The figure shows three views and two pictorial views of one solid part (mm, origin at its lowest corner). Answer the questions. Give positions to 0.01 mm unless a question says otherwise; leave off trailing zeros. Loops run counter-clockwise (first coordinate to the right, second up) from the corner with the lowest first, then second, coordinate; pieces in that order, holes last. Notation, with made-up numbers: M -14.75,53 L 20.25,53 A25 ccw 20.25,71 Z; hole C 0.5,74.25 d7. An arc over 180 degrees is marked long. Answer as a JSON object with one key per item and string values. Group by question number.
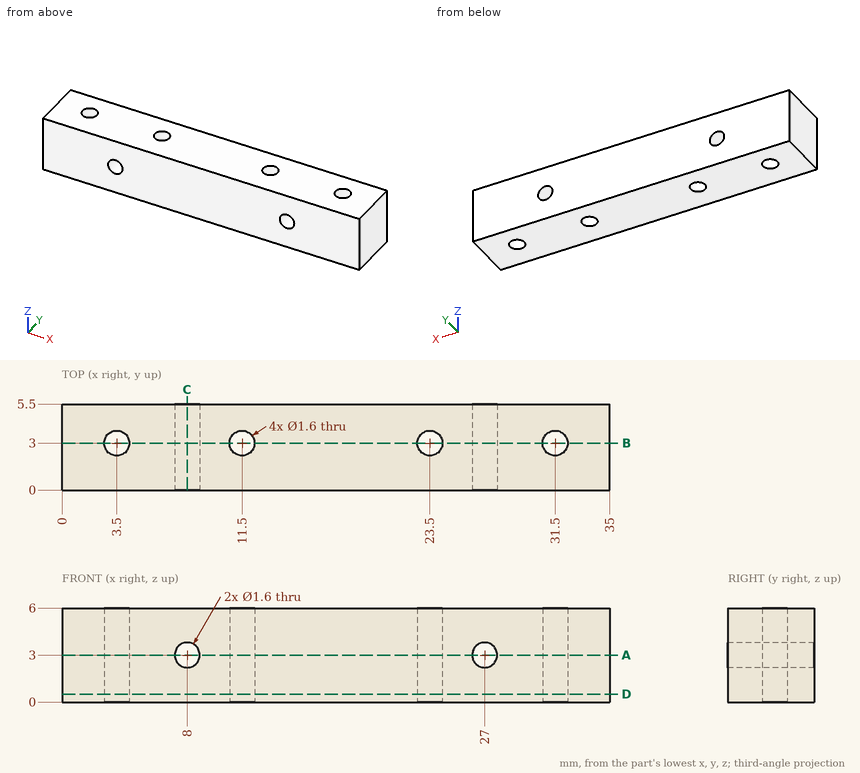
Item 1: A cutting plane is placed at C-C (x = 8). Determine the outline of the cut face in (y, z), and give its area (3 significant figures).
Item 2: Find the intervals of material crossed by probe 1 along Y at (x, z) = (3.5, 4.45); probe 2 along Z at (x, y) = (8, 4.45); probe 3 along X at (y, z) = (0.55, 3.1), in increasing order. Write a range as [from, to].
Item 3: A cutting plane is placed at D-D (z = 0.5). Determine the outline of the cut face in (x, y), and give its area (3 significant figures).
Item 4: A cutting plane is placed at B-B (y = 3). Determine the outline of the cut face in (x, z), and give its area (3 significant figures).
Item 5: A cutting plane is placed at A-A (z = 3). Determine the outline of the cut face in (x, y).
The answers:
{
 "1": {"outline": "M 0,0 L 5.5,0 L 5.5,2.2 L 0,2.2 Z; M 0,3.8 L 5.5,3.8 L 5.5,6 L 0,6 Z", "area": "24.2 mm^2"},
 "2": {"probe 1": "y = [0, 2.2], [3.8, 5.5]", "probe 2": "z = [0, 2.2], [3.8, 6]", "probe 3": "x = [0, 7.21], [8.79, 26.21], [27.79, 35]"},
 "3": {"outline": "M 0,0 L 35,0 L 35,5.5 L 0,5.5 Z; hole C 3.5,3 d1.6; hole C 11.5,3 d1.6; hole C 23.5,3 d1.6; hole C 31.5,3 d1.6", "area": "184 mm^2"},
 "4": {"outline": "M 0,0 L 2.7,0 L 2.7,6 L 0,6 Z; M 4.3,0 L 10.7,0 L 10.7,6 L 4.3,6 Z; M 12.3,0 L 22.7,0 L 22.7,6 L 12.3,6 Z; M 24.3,0 L 30.7,0 L 30.7,6 L 24.3,6 Z; M 32.3,0 L 35,0 L 35,6 L 32.3,6 Z; hole C 8,3 d1.6; hole C 27,3 d1.6", "area": "168 mm^2"},
 "5": {"outline": "M 0,0 L 7.2,0 L 7.2,5.5 L 0,5.5 Z; M 8.8,0 L 26.2,0 L 26.2,5.5 L 8.8,5.5 Z; M 27.8,0 L 35,0 L 35,5.5 L 27.8,5.5 Z; hole C 3.5,3 d1.6; hole C 11.5,3 d1.6; hole C 23.5,3 d1.6; hole C 31.5,3 d1.6"}
}
